The listing builds one solid part. Answer for the finished solid, in the listing's coordinates (mm). A direction names the side the tool comes from. Coordinates: 2 decimals unless noted, no trailing zeros. Order: outer loops, then holes, each group sorted by start corner. A loop starts at its lowest first (then second) coordinate and runs counter-clockwise, first axis right, second up. Notation, with made-up numbers: (69, -38.75) -> (117, -38.75) arc R23 cw to (117, -4.75) -> close; hole circle Ø1 at (-33.75, 57). An arc over 180 degrees is marked (long way). One line per question, with ' | ' between items.
from build123d import *

# Parameters (mm, degrees)
F0_W      = 109.3159876764
F0_H      = 56.5186925232
F1_DEPTH  = 25.4
F2_W      = 55.8209288865
F2_H      = 56.5186925232
F3_DEPTH  = 27.94
F4_W      = 23.2587223873
F4_H      = 23.4913080931
F5_DEPTH  = 43.18
F7_DEPTH  = 25.4
F8_DEPTH  = 38.1
F10_DEPTH = 58.42
F12_DEPTH = 25.4
F14_D     = 11.43
F16_D     = 11.43


with BuildPart() as f1:
    # F0 (on Top) → F1 (new body)
    with BuildSketch(Plane.XY):
        with Locations((0.3488790244, 4.7680381685)):
            Rectangle(F0_W, F0_H)
    extrude(amount=F1_DEPTH)

    # F2 (on face) → F3 (join)
    with BuildSketch(Plane.XY.offset(25.4)):
        with Locations((0.1162933186, 4.7680381685)):
            Rectangle(F2_W, F2_H)
    extrude(amount=F3_DEPTH)

    # F4 (on face) → F5 (cut)
    with BuildSketch(Plane.XY.offset(53.34)):
        with Locations((-0.5814679898, -11.7456540465)):
            Rectangle(F4_W, F4_H)
    extrude(amount=-F5_DEPTH, mode=Mode.SUBTRACT)

    # F6 (on face) → F7 (cut)
    with BuildSketch(Plane.XZ.offset(23.4913080931)):
        Polygon((-27.7941711247, 25.4), (-20.0025001541, 53.34), (-27.7941711247, 53.34), align=None)
    extrude(amount=-F7_DEPTH, mode=Mode.SUBTRACT)

    # F8 (cut): a face of the model
    f8_faces = [f1.faces().sort_by_distance(p)[0] for p in [
        (-25.1969474678, 1.9086919069, 44.0266666667),
    ]]
    extrude(f8_faces, amount=-F8_DEPTH, mode=Mode.SUBTRACT)

    # F9 (on face) → F10 (cut)
    with BuildSketch(Plane.XZ.offset(23.4913080931)):
        Polygon((28.0267577618, 53.34), (19.5373254828, 53.34), (28.0267577618, 25.4), align=None)
    extrude(amount=-F10_DEPTH, mode=Mode.SUBTRACT)

    # F11 (on face) → F12 (join)
    with BuildSketch(Plane.YZ.offset(-12.2108291835)):
        Polygon((0, 10.16), (0, 53.34), (-23.4913080931, 10.16), align=None)
    extrude(amount=F12_DEPTH)

    # F14 (through all)
    with Locations(Plane.XY.offset(25.4)):
        with Locations((-42.5856821239, 4.861375317)):
            Hole(F14_D / 2)

    # F16 (through all)
    with Locations(Plane.XY.offset(25.4)):
        with Locations((41.6108891368, 4.2035188526)):
            Hole(F16_D / 2)


solid = f1.part
Item 1: Section A-A, the plane y = 29 is taken. Give the vertices of the cut face in (x, z), plus the area to 3 significant figures.
Computed values:
outline: (-54.31, 0) -> (55.01, 0) -> (55.01, 25.4) -> (28.03, 25.4) -> (19.54, 53.34) -> (-20, 53.34) -> (-27.79, 25.4) -> (-54.31, 25.4) -> close | area: 4,110 mm^2
Item 2: Section B-B, the plane z = 24 is taken. Give the vertices of the cut face in (x, y) (3 decimals).
Computed values:
outline: (-54.309, -23.491) -> (-12.211, -23.491) -> (-12.211, -15.962) -> (11.048, -15.962) -> (11.048, -23.491) -> (55.007, -23.491) -> (55.007, 33.027) -> (-54.309, 33.027) -> close; hole circle Ø11.43 at (-42.586, 4.861); hole circle Ø11.43 at (41.611, 4.204)
Item 3: Section D-D, the plane x = -4 is taken. Give the vertices of the cut face in (y, z).
Computed values:
outline: (-23.49, 0) -> (33.03, 0) -> (33.03, 53.34) -> (0, 53.34) -> (-23.49, 10.16) -> close
Item 4: Determine the mould class of faces 4 (the face through (-54.309, 4, 13)), 5 (the face through (35, 5, 25.4)), 6 (the face through (55.007, 4, 13)), 7 (the face through (36.16, 5.92, 12.52)) for opening direction X: pulls with the +X half, pulls with the -X half, needs draft (parallel to the pull), parting line crosses it, or undercut.
Computed values:
face 4: pulls with the -X half | face 5: needs draft | face 6: pulls with the +X half | face 7: undercut
Item 5: For faces 1 (the face through (23.72, 4.37, 39.57)), 2 (the face through (-35, 5, 25.4)), 3 (the face through (-12.211, -15, 37)), determine the directions among +Z, -Z, +X, -X, +Y, -Y from which every point of the face is accessible in a straight line to the end or side of a thin tool.
Computed values:
face 1: +Z, +X, +Y, -Y | face 2: +Z, -X, +Y, -Y | face 3: +Z, -Y
Item 6: Each of these flat-tipped pins is pushed along its axis until it touches: pin 1 Ø7 at (x, y) = (-42.59, 4.86) entering from -Z; pin 2 Ø5 at (x, y) = (0, -11.5) entering from +Z; pin 3 Ø1.5 at (y, z) = (16, 30.5) entering from -X; pin 4 Ø10 at (y, z) = (14.5, 36) entering from +X. Where does it stop, or does it pass through?
Computed values:
pin 1: passes through | pin 2: stops at z = 36.8 | pin 3: stops at x = -26.58 | pin 4: stops at x = 26.33
Item 7: Section C-C, the plane y = 7.5 is taken. Give the vertices of the cut face in (x, z), plus the area to 3 significant figures.
Computed values:
outline: (-54.31, 0) -> (-47.66, 0) -> (-47.66, 25.4) -> (-54.31, 25.4) -> close; (-37.52, 0) -> (36.94, 0) -> (36.94, 25.4) -> (28.03, 25.4) -> (19.54, 53.34) -> (-20, 53.34) -> (-27.79, 25.4) -> (-37.52, 25.4) -> close; (46.28, 0) -> (55.01, 0) -> (55.01, 25.4) -> (46.28, 25.4) -> close | area: 3,610 mm^2
Item 8: Find the intervals of material crossed by L1, parallel to X at y = 5, z = 24; L2, parallel to Z at x = 38.5, y = 20.5; L3, parallel to X at y = -8.5, z = 42.5, in increasing order.
Computed values:
L1: x = -54.31 to -48.3, -36.87 to 35.95, 47.27 to 55.01 | L2: z = 0 to 25.4 | L3: x = -23.03 to -12.21, 11.05 to 22.83
